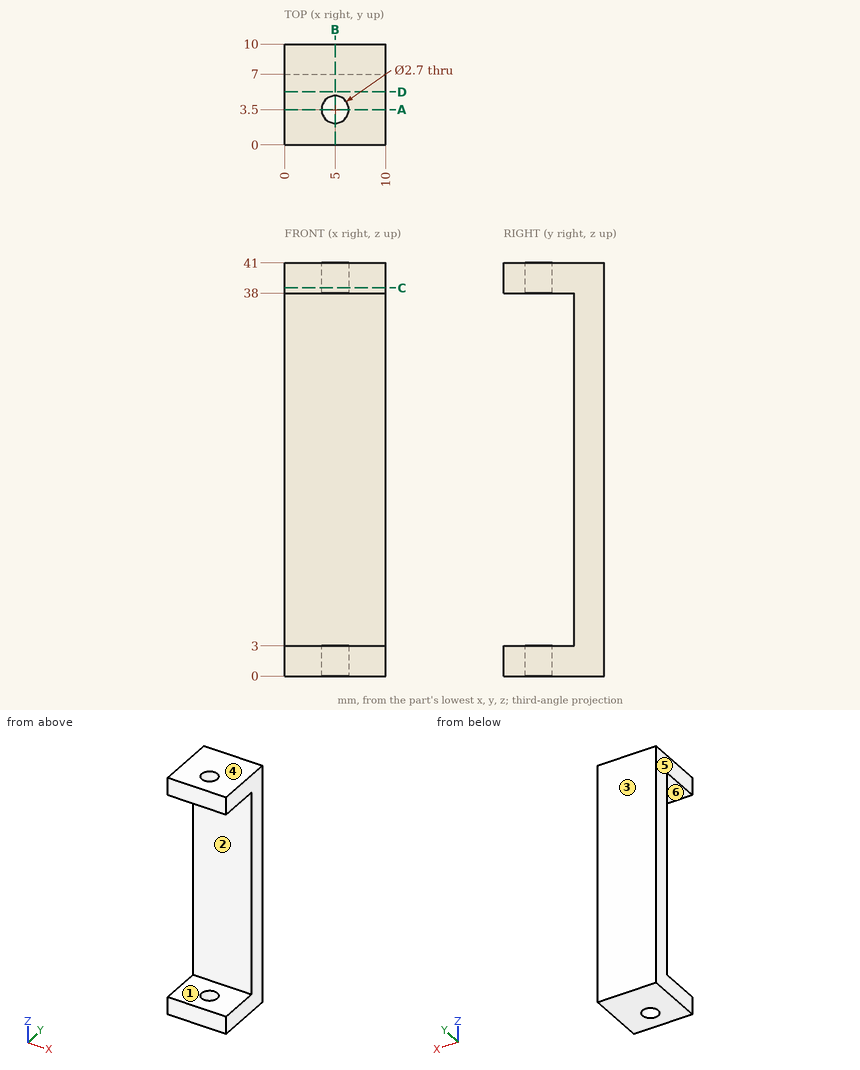
Input: dimensioned drawing with shaded views. Units: mm. Origin: part minimum x, y, z. A direction names the side the tool comes from. Round coordinates to 2 decimals unless told otherwise and drop trailing zeros. Order: outer loops, then holes, each group sorted by start corner. A loop starts at its lowest first (then second) coordinate and runs counter-clockwise, first axis right, second up. Notation, with made-up numbers: (61, 62) - (91, 62) arc R25 ccw to (91, 75) - close; hole circle Ø2 at (-39.5, 15.5). An arc over 180 degrees is marked (long way). Answer as a JSON object with one key per item and string values. Group by question number.
(1) Pin query (flat end, axial travel): P1, Ø3, axis at x = 4, z = 19, coming from the -Y side; P2, Ø1.6, axis at x = 5, y = 3.5, coming from the +Z side. Return the tip coordinate at first contact, or that it passes through.
(2) Draft query along Z for the marked faces 1, 2, 3 and 4. Return one class per face: released by +Z, released by -Z, zero draft, split by the parting line, or undercut.
(3) Reachability of the marked faces 5 and 6 from +Z, -Z, +X, -X, +Y, -Y: full face, straight path, thin tool, end or side. Return the list, or none.
(4) Cut plane D-D (y = 5.25). Return loops of the section in (x, z), then the cut area to 3 significant figures.
(5) Material intervals for probe 1 along Z at (x, y) = (3.5, 5.75); probe 2 along Y at (x, z) = (5, 40.05); probe 3 along Y at (x, z) = (5.25, 12), sorted ascending. Write a range as from..to.
(6) Cut plane B-B (x = 5). Return loops of the section in (y, z).
(7) Cut plane A-A (y = 3.5). Return loops of the section in (x, z).
(8) Cut plane C-C (z = 38.5). Return loops of the section in (x, y).
Here are the results:
{
 "1": {"P1": "stops at y = 7", "P2": "passes through"},
 "2": {"face 1": "undercut", "face 2": "undercut", "face 3": "zero draft", "face 4": "released by +Z"},
 "3": {"face 5": "+Z, -Z, -X, +Y, -Y", "face 6": "+X, -X, -Y"},
 "4": {"outline": "(0, 0) - (10, 0) - (10, 3) - (0, 3) - close; (0, 38) - (10, 38) - (10, 41) - (0, 41) - close", "area": "60.0 mm^2"},
 "5": {"probe 1": "z = 0..3, 38..41", "probe 2": "y = 0..2.15, 4.85..10", "probe 3": "y = 7..10"},
 "6": {"outline": "(0, 0) - (2.15, 0) - (2.15, 3) - (0, 3) - close; (0, 38) - (2.15, 38) - (2.15, 41) - (0, 41) - close; (4.85, 0) - (10, 0) - (10, 41) - (4.85, 41) - (4.85, 38) - (7, 38) - (7, 3) - (4.85, 3) - close"},
 "7": {"outline": "(0, 0) - (3.65, 0) - (3.65, 3) - (0, 3) - close; (0, 38) - (3.65, 38) - (3.65, 41) - (0, 41) - close; (6.35, 0) - (10, 0) - (10, 3) - (6.35, 3) - close; (6.35, 38) - (10, 38) - (10, 41) - (6.35, 41) - close"},
 "8": {"outline": "(0, 0) - (10, 0) - (10, 10) - (0, 10) - close; hole circle Ø2.7 at (5, 3.5)"}
}
